Verification items for the finished model (mm, model axes). Face numbers are marked on the shaded views. A direction names the side the tool comes from. Give positions to 0.01 mm unless a question says otherwise; leave off trailing zeros. Order: outer loops, then holes, each group sorted by start corner. A loop starts at its lowest first (then second) coordinate and runs counter-clockwise, first axis right, second up. Notation, with made-up numbers: (-33.5, 71) - (23.5, 71) arc R13 ccw to (23.5, 83) - close; hole circle Ø3 at (83, 52). An arc over 180 degrees is marked (long way). Answer as a JSON object with one key per item and string values.
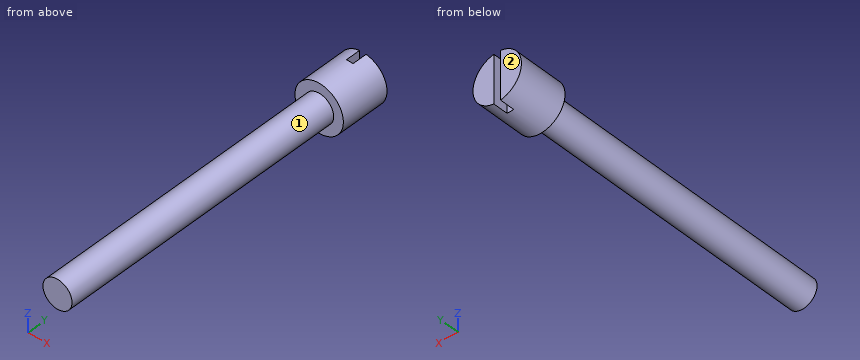
```python
from build123d import *

# Parameters (mm, degrees)
F0_R     = 3
F1_DEPTH = 60
F2_R     = 5
F3_DEPTH = 10
F4_W     = 1.377778
F4_H     = 10
F5_DEPTH = 3


with BuildPart() as f1:
    # F0 (on Front) → F1 (new body)
    with BuildSketch(Plane.XZ):
        Circle(F0_R)
    extrude(amount=F1_DEPTH)

    # F2 (on Front) → F3 (join)
    with BuildSketch(Plane.XZ):
        Circle(F2_R)
    extrude(amount=-F3_DEPTH)

    # F4 (on face) → F5 (cut)
    with BuildSketch(Plane(origin=(0, 10, 0), x_dir=(-1, 0, 0), z_dir=(0, 1, 0))):
        Rectangle(F4_W, F4_H)
    extrude(amount=-F5_DEPTH, mode=Mode.SUBTRACT)


solid = f1.part
```
(1) Section check C-C (y = 6). Record the cut outline in (x, z).
Computed values:
{"outline": "circle Ø10 at (0, 0)"}
(2) Section check A-A (x = 0). Record the cut outline in (y, z), then the cut area to 3 significant figures.
Computed values:
{"outline": "(-60, -3) - (0, -3) - (0, -5) - (7, -5) - (7, 5) - (0, 5) - (0, 3) - (-60, 3) - close", "area": "430 mm²"}
(3) Gauge pin test, flat ends, axial feed: pin 1 Ø4 at (x, y) = (3.5, -33) entering from +Z; pin 2 Ø1.1 at (x, z) = (0, -1) entering from +Y; pin 3 Ø2.5 at (y, z) = (8, 2.5) entering from -X. Record the tip position at first contact, or that the pin passes through.
Computed values:
{"pin 1": "stops at z = 2.6", "pin 2": "stops at y = 7", "pin 3": "stops at x = -4.84"}
(4) Material ranges on line 1 along Y through (x, z) = (-2, 3.25); line 2 along Y through (x, z) = (0, 3.75); line 3 along Z through (x, y) = (-0.75, -54.5), recorded low to high. Write a range as [from, to].
Computed values:
{"line 1": "y = [0, 10]", "line 2": "y = [0, 7]", "line 3": "z = [-2.9, 2.9]"}
(5) Section check B-B (z = 0). Record the cut outline in (x, y), then the cut area to 3 significant figures.
Computed values:
{"outline": "(-5, 0) - (-3, 0) - (-3, -60) - (3, -60) - (3, 0) - (5, 0) - (5, 10) - (0.69, 10) - (0.69, 7) - (-0.69, 7) - (-0.69, 10) - (-5, 10) - close", "area": "456 mm²"}
(6) Access from +Z, -Z, +X, -X, +Y, -Y to the whole of each face (thin tool, end or side, straight path). Record for the marked faces 1 and 2.
Computed values:
{"face 1": "-Y", "face 2": "+Z, -Z, +X, -X, +Y"}
(7) Section check D-D (z = -3.75). Record the cut outline in (x, y).
Computed values:
{"outline": "(-3.31, 0) - (3.31, 0) - (3.31, 10) - (0.69, 10) - (0.69, 7) - (-0.69, 7) - (-0.69, 10) - (-3.31, 10) - close"}
